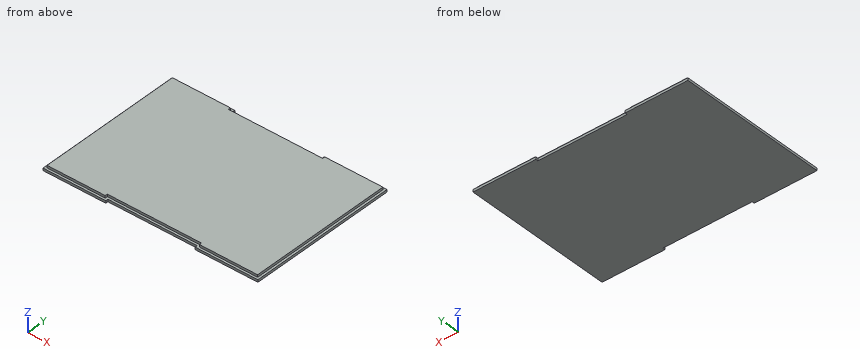
from build123d import *

# Parameters (mm, degrees)
F0_W     = 26
F0_H     = 1
F0_H_2   = 60
F0_W_2   = 37
F1_DEPTH = 1
F2_W     = 39
F2_H     = 58.2
F3_DEPTH = 1


with BuildPart() as f1:
    # F0 (on Top) → F1 (new body)
    with BuildSketch(Plane.XY):
        with Locations((31.5, -30.5)):
            Rectangle(F0_W, F0_H)
        with Locations((31.5, 0)):
            Rectangle(F0_W, F0_H_2)
        Rectangle(F0_W_2, F0_H_2)
        with Locations((31.5, 30.5)):
            Rectangle(F0_W, F0_H)
        with Locations((-31.5, -30.5)):
            Rectangle(F0_W, F0_H)
        with Locations((-31.5, 0)):
            Rectangle(F0_W, F0_H_2)
        with Locations((-31.5, 30.5)):
            Rectangle(F0_W, F0_H)
    extrude(amount=F1_DEPTH)

    # F2 (on face) → F3 (join)
    with BuildSketch(Plane.XY.offset(1)):
        Polygon((-19.5, 30.1), (-43.6, 30.1), (-43.6, -30.1), (-19.5, -30.1), (-19.5, -29.1), (-19.5, 29.1), align=None)
        Rectangle(F2_W, F2_H)
        Polygon((19.5, 30.1), (19.5, 29.1), (19.5, -29.1), (19.5, -30.1), (43.6, -30.1), (43.6, 30.1), align=None)
    extrude(amount=F3_DEPTH)


solid = f1.part
Geometry: final body of the model. Coordinates: model frame, mm. Give positions to 0.01 mm unless a question says otherwise; leave off trailing zeros. Order: outer loops, then holes, each group sorted by start corner. A loop starts at its lowest first (then second) coordinate and runs counter-clockwise, first axis right, second up. Notation, with made-up numbers: (57.5, -25) -> (79.5, -25) arc R23 cw to (79.5, 13) -> close; hole circle Ø10 at (64.25, 28). An arc over 180 degrees is marked (long way). Answer as a JSON object with one key per item and string values.
Q1. Section B-B (x = -9.5). Output: boundary loops of the cut face in (y, z), plus the area to 3 significant figures.
Entries:
{"outline": "(-30, 0) -> (30, 0) -> (30, 1) -> (29.1, 1) -> (29.1, 2) -> (-29.1, 2) -> (-29.1, 1) -> (-30, 1) -> close", "area": "118 mm^2"}
Q2. First-contact query: pin 1 (0.8 mm diameter, centred on y = -30, z = 1.5, fed in from +X); pin 2 (0.8 mm diameter, centred on x = 32.5, z = 1.5, fed in from -Y); pin 3 (0.5 mm diameter, centred on x = -6.5, z = 1.5, fed in from -Y). Flat tips, straight axial feed; report the tip coordinate or a pass-through.
Entries:
{"pin 1": "stops at x = 43.6", "pin 2": "stops at y = -30.1", "pin 3": "stops at y = -29.1"}
Q3. Material intervals for probe 1 along Y at (x, z) = (-15.5, 1.3); probe 2 along Y at (x, z) = (-14, 0.9); probe 3 along X at (y, z) = (6, 1.05), sorted ascending.
Entries:
{"probe 1": "y = -29.1 to 29.1", "probe 2": "y = -30 to 30", "probe 3": "x = -43.6 to 43.6"}
Q4. Section A-A (z = 1.45). Output: boundary loops of the cut face in (x, y), plus the area to 3 significant figures.
Entries:
{"outline": "(-43.6, -30.1) -> (-19.5, -30.1) -> (-19.5, -29.1) -> (19.5, -29.1) -> (19.5, -30.1) -> (43.6, -30.1) -> (43.6, 30.1) -> (19.5, 30.1) -> (19.5, 29.1) -> (-19.5, 29.1) -> (-19.5, 30.1) -> (-43.6, 30.1) -> close", "area": "5,170 mm^2"}
